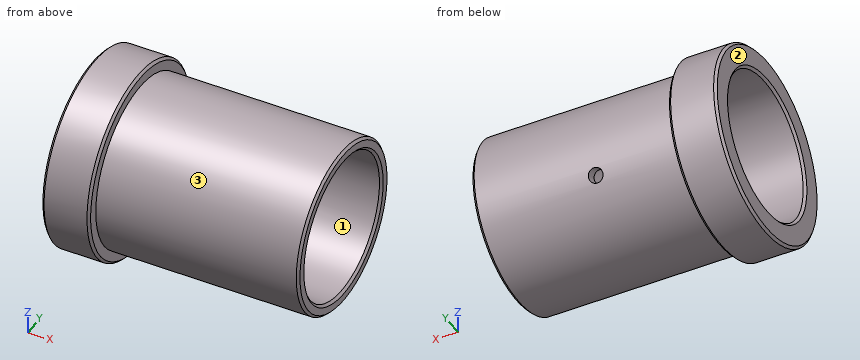
```python
from build123d import *

# Parameters (mm, degrees)
CHAMFER_1_SIZE           = 1
SKETCH_2_R               = 3
CUT_EXTRUDE_1_DEPTH      = 10
CUT_EXTRUDE_1_DEPTH_BACK = 108


with BuildPart() as part:
    # Эскиз1 → Повернуть1 (revolve)
    with BuildSketch(Plane.XY):
        Polygon((0, 40), (0, 30), (105, 30), (105, 35), (20, 35), (20, 40), align=None)
    revolve(axis=Axis((0, 0, 0), (1, 0, 0)))

    # Фаска1
    chamfer_1_edges = [part.edges().sort_by_distance(p)[0] for p in [
        (20, -40, 0),
        (105, -35, 0),
        (105, -30, 0),
        (0, -30, 0),
        (0, -40, 0),
    ]]
    chamfer(chamfer_1_edges, length=CHAMFER_1_SIZE)

    # Эскиз2 → Вырез-Вытянуть1 (cut, two sides)
    with BuildSketch(Plane(origin=(110, 102, -50), x_dir=(1, 0, 0), z_dir=(0, 0.897920723, -0.440157217))) as cut_extrude_1_sk:
        with Locations((-55, 0)):
            Circle(SKETCH_2_R)
    extrude(amount=CUT_EXTRUDE_1_DEPTH, mode=Mode.SUBTRACT)
    extrude(cut_extrude_1_sk.sketch, amount=-CUT_EXTRUDE_1_DEPTH_BACK, mode=Mode.SUBTRACT)


solid = part.part
```
Check sheet for the modelled part. Datum: model origin and axes. Units: mm. Face numbers are marked on the shaded views. Round coordinates to 2 decimals unless told otherwise and drop trailing zeros. Order: outer loops, then holes, each group sorted by start corner. A loop starts at its lowest first (then second) coordinate and runs counter-clockwise, first axis right, second up. Notation, with made-up numbers: (29, -27) -> (34, -27) arc R17 ccw to (34, 3) -> close; hole circle Ø7 at (-26.75, -8). An arc over 180 degrees is marked (long way). One line per item, written item: value. Start each with the question number.
Q1. Mould release check, pull along Z, two halves, no side actions. Record for the marked faces 1, 2 and 3: pulls with the +Z half, pulls with the -Z half, needs draft (parallel to the pull), parting line crosses it, or undercut.
Q2. Cross-section at C-C (x = 48.5). Record the boundary of the cut face in (y, z), and give its area (3 significant figures).
Q3. Thickness scan on line 1 (Z direction, x = 32.5, y = 0); line 2 (X direction, y = -5.5, z = 35.5); line 3 (Z direction, x = 9, y = 24.5). Record the ranges inside material, lowest first.
Q4. Cross-section at A-A (y = 0). Record the boundary of the cut face in (x, z), and give its area (4 significant figures).
Q5. Gauge pin test, flat ends, axial feed: pin 1 Ø23.5 at (y, z) = (-7, 10) entering from +X; pin 2 Ø4 at (x, z) = (78, 25) entering from -Y; pin 3 Ø4 at (x, y) = (51, -25) entering from +Z; pin 4 Ø4 at (x, y) = (91.5, -18) entering from +Z. Record the tip position at first contact, or that the pin passes through.
Completed:
1. face 1: undercut
1. face 2: needs draft
1. face 3: parting line crosses it
2. outline: circle Ø70 at (0, 0); hole circle Ø60 at (0, 0)
2. area: 1,020 mm²
3. line 1: z = -35 to -30, 30 to 35
3. line 2: x = 0 to 20
3. line 3: z = -31.62 to -17.31, 17.31 to 31.62
4. outline: (0, -39) -> (1, -40) -> (19, -40) -> (20, -39) -> (20, -35) -> (104, -35) -> (105, -34) -> (105, -31) -> (104, -30) -> (1, -30) -> (0, -31) -> close; (0, 31) -> (1, 30) -> (104, 30) -> (105, 31) -> (105, 34) -> (104, 35) -> (20, 35) -> (20, 39) -> (19, 40) -> (1, 40) -> (0, 39) -> close
4. area: 1,245 mm²
5. pin 1: passes through
5. pin 2: stops at y = -26.38
5. pin 3: stops at z = 26.38
5. pin 4: stops at z = 31.13
